For this review, take the finished solid that the model builds, in its own axes (mm). A direction names the side the tool comes from. Round coordinates to 2 decimals unless told otherwise and drop trailing zeros. Loops run counter-clockwise (first coordinate to the right, second up) from the corner with the lowest first, then second, coordinate; pieces in that order, holes last.
1) Insertion check: pin 1 (1 mm diameter, centred on x = 307.5, y = -24, fed in from -Z); pin 2 (2 mm diameter, centred on x = 79.5, y = -113.5, fed in from +Z); pin 3 (2 mm diameter, centred on x = 195.5, y = 26.5, fed in from -Z). Each pin has a flat end and moves straight along its axis. Give the tip position at first contact, or say it passes through.
2) Take a section at C-C (x = 143). State the section outline as (y, z) points.
3) Take a section at B-B (z = -29.5). State the section outline as (x, y) points.
4) Take a section at D-D (y = 214.5). State the section outline as (x, z) points.
5) Take a section at A-A (y = -44.5). State the section outline as (x, z) points.
6) Wall thickness on L1, parallel to Y at x = 10, z = -0.6; L2, parallel to Z at x = 200, y = -121; L3, parallel to Z at x = 321.5, y = 176: over which ranges is each line inside the solid? List them lowest first.
7) Tool access review of faces 1 (the flat face through (10, -4, -2)), 2 (the flat face through (187.451, -3.779, -24.367)): name each direction out of +Z, -Z, +X, -X, +Y, -Y from which nothing blocks a thin tool from reaching the whole face with its end or side.
```python
from build123d import *

# Parameters (mm, degrees)
F1_DEPTH = 270
F3_DEPTH = 55
F4_R     = 4
F5_R     = 2
F6_R     = 5
F7_R     = 3.25
F8_DEPTH = 25


with BuildPart() as f1:
    # F0 (on Front) → F1 (new body, symmetric)
    with BuildSketch(Plane.XZ):
        Polygon((20, 0), (0, 0), (0, -2), (19.855245, -2), (349.711998, -50), (350, -48.020845), align=None)
    extrude(amount=F1_DEPTH, both=True)

    # F2 (on face) → F3 (cut)
    with BuildSketch(Plane.XY):
        Polygon((350, -200), (20, -270), (20, -308.046314), (437.196553, -308.046314), (437.196553, -200), align=None)
        Polygon((20, 308.046314), (20, 270), (350, 200), (437.196553, 200), (437.196553, 308.046314), align=None)
    extrude(amount=-F3_DEPTH, mode=Mode.SUBTRACT)

    # F4
    f4_edges = [f1.edges().sort_by_distance(p)[0] for p in [
        (20, 0, 0),
    ]]
    fillet(f4_edges, radius=F4_R)

    # F5
    f5_edges = [f1.edges().sort_by_distance(p)[0] for p in [
        (19.855245, 0, -2),
    ]]
    fillet(f5_edges, radius=F5_R)

    # F6
    f6_edges = [f1.edges().sort_by_distance(p)[0] for p in [
        (349.855999, -200.030546, -49.010422),
        (349.855999, 200.030546, -49.010422),
    ]]
    fillet(f6_edges, radius=F6_R)

    # F7 (on face) → F8 (cut)
    with BuildSketch(Plane.XY):
        with Locations((10, 0)):
            Circle(F7_R)
    extrude(amount=-F8_DEPTH, mode=Mode.SUBTRACT)


solid = f1.part
```
Response:
1. pin 1: stops at z = -43.93
1. pin 2: stops at z = -8.51
1. pin 3: stops at z = -27.7
2. outline: (-243.91, -19.92) - (243.91, -19.92) - (243.91, -17.9) - (-243.91, -17.9) - close
3. outline: (208.84, -229.94) - (222.72, -227) - (222.72, 227) - (208.84, 229.94) - close
4. outline: (0, -2) - (19.71, -2) arc R2 cw to (20, -2.02) - (281.64, -40.09) - (281.64, -38.07) - (20.29, -0.04) arc R4 ccw to (19.71, 0) - (0, 0) - close
5. outline: (0, -2) - (19.71, -2) arc R2 cw to (20, -2.02) - (349.71, -50) - (350, -48.02) - (20.29, -0.04) arc R4 ccw to (19.71, 0) - (0, 0) - close
6. L1: y = -270 to -3.25, 3.25 to 270
6. L2: z = -28.21 to -26.19
6. L3: z = -45.89 to -43.87
7. face 1: -Z, -X, +Y, -Y
7. face 2: +Z, +X, +Y, -Y
